```python
from build123d import *

# Parameters (mm, degrees)
SKETCH1_R            = 15
BOSS_EXTRUDE1_DEPTH  = 30
SKETCH8_W            = 30
SKETCH8_H            = 15
REVOLVE1_ANGLE       = 180
SKETCH9_W            = 30
SKETCH9_H            = 30
BOSS_EXTRUDE3_DEPTH  = 15
SKETCH10_R           = 5
CUT_EXTRUDE1_DEPTH   = 30
SKETCH13_R           = 16
CUT_EXTRUDE2_DEPTH   = 10
SKETCH14_W           = 10
SKETCH14_H           = 15
CUT_EXTRUDE3_DEPTH   = 67
CUT_EXTRUDE4_START   = -7
SKETCH15_R           = 11
SKETCH15_R_2         = 5
CUT_EXTRUDE4_DEPTH   = 7
SKETCH16_R           = 11
SKETCH16_R_2         = 5
CUT_EXTRUDE5_DEPTH   = 7
SKETCH17_R           = 15
SKETCH17_R_2         = 8
SKETCH17_R_3         = 3.5
BOSS_EXTRUDE4_DEPTH  = 2
BOSS_EXTRUDE5_DEPTH  = 5
BOSS_EXTRUDE6_DEPTH  = 16
SKETCH21_W           = 53
SKETCH21_H           = 30
CUT_EXTRUDE7_DEPTH   = 20
SKETCH23_W           = 15
SKETCH23_H           = 9
SKETCH24_W           = 30
SKETCH24_H           = 9
BOSS_EXTRUDE7_DEPTH  = 15
SKETCH25_R           = 4
CUT_EXTRUDE8_DEPTH   = 15
BOSS_EXTRUDE8_START  = 3
SKETCH26_W           = 10
SKETCH26_H           = 15
BOSS_EXTRUDE8_DEPTH  = 5
SKETCH30_W           = 30
SKETCH30_H           = 15
BOSS_EXTRUDE9_DEPTH  = 3
SKETCH27_R           = 16
CUT_EXTRUDE9_DEPTH   = 16
SKETCH28_R           = 16
CUT_EXTRUDE10_DEPTH  = 10.5
SKETCH29_R           = 16
CUT_EXTRUDE12_DEPTH  = 10
SKETCH31_W           = 53
SKETCH31_H           = 41.496728026
CUT_EXTRUDE13_DEPTH  = 37
BOSS_EXTRUDE10_DEPTH = 5
SKETCH35_W           = 30
SKETCH35_H           = 9
BOSS_EXTRUDE11_DEPTH = 5
SKETCH36_R           = 16
CUT_EXTRUDE14_DEPTH  = 13.5
SKETCH37_R           = 16
CUT_EXTRUDE15_DEPTH  = 18.5
FILLET1_R            = 5


with BuildPart() as part:
    # Sketch1 → Boss-Extrude1 (new body)
    with BuildSketch(Plane(origin=(0, 0, 0), x_dir=(1, 0, 0), z_dir=(0, 1, 0))):
        with Locations(Location((0, 0, 0), (0, 0, 270))):
            Circle(SKETCH1_R)
    extrude(amount=BOSS_EXTRUDE1_DEPTH)

    # Sketch8 → Revolve1 (revolve)
    with BuildSketch(Plane(origin=(0, 30, 0), x_dir=(1, 0, 0), z_dir=(0, 1, 0))):
        with Locations((0, -7.5)):
            Rectangle(SKETCH8_W, SKETCH8_H)
    revolve(axis=Axis((15, 30, 0), (-1, 0, 0)), revolution_arc=REVOLVE1_ANGLE)

    # Sketch9 → Boss-Extrude3 (add)
    with BuildSketch(Plane.XZ.offset(-30)):
        Rectangle(SKETCH9_W, SKETCH9_H)
    extrude(amount=BOSS_EXTRUDE3_DEPTH)

    # Sketch10 → Cut-Extrude1 (cut)
    with BuildSketch(Plane(origin=(15, 0, 0), x_dir=(0, 0, -1), z_dir=(1, 0, 0))):
        with Locations((0, 30)):
            Circle(SKETCH10_R)
    extrude(amount=-CUT_EXTRUDE1_DEPTH, mode=Mode.SUBTRACT)

    # Sketch13 → Cut-Extrude2 (cut)
    with BuildSketch(Plane(origin=(5, 0, 0), x_dir=(0, 0, -1), z_dir=(1, 0, 0))):
        with Locations((0, 30)):
            Circle(SKETCH13_R)
    extrude(amount=-CUT_EXTRUDE2_DEPTH, mode=Mode.SUBTRACT)

    # Sketch14 → Cut-Extrude3 (cut)
    with BuildSketch(Plane.XY.offset(15)):
        with Locations((0, 22.5)):
            Rectangle(SKETCH14_W, SKETCH14_H)
    extrude(amount=-CUT_EXTRUDE3_DEPTH, mode=Mode.SUBTRACT)

    # Sketch15 → Cut-Extrude4 (cut)
    with BuildSketch(Plane.ZY.offset(15).offset(CUT_EXTRUDE4_START)):
        with Locations((0, 30)):
            Circle(SKETCH15_R)
        with Locations(Location((0, 30, 0), (0, 0, 180))):
            Circle(SKETCH15_R_2, mode=Mode.SUBTRACT)
    extrude(amount=CUT_EXTRUDE4_DEPTH, mode=Mode.SUBTRACT)

    # Sketch16 → Cut-Extrude5 (cut)
    with BuildSketch(Plane(origin=(15, 0, 0), x_dir=(0, 0, -1), z_dir=(1, 0, 0))):
        with Locations(Location((0, 30, 0), (0, 0, 180))):
            Circle(SKETCH16_R)
        with Locations((0, 30)):
            Circle(SKETCH16_R_2, mode=Mode.SUBTRACT)
    extrude(amount=-CUT_EXTRUDE5_DEPTH, mode=Mode.SUBTRACT)



with BuildPart() as body_2:
    # Sketch17 → Boss-Extrude4 (new body)
    # profile 1 of 4: a face of its own
    with BuildSketch(Plane.ZY.offset(31)):
        with Locations((0, 30)):
            Circle(SKETCH17_R)
        with Locations((0, 30)):
            Circle(SKETCH17_R_2, mode=Mode.SUBTRACT)
    # profile 2 of 4: a face of its own
    with BuildSketch(Plane.ZY.offset(31)):
        with Locations((0, 30)):
            Circle(SKETCH17_R_2)
        with Locations((0, 30)):
            Circle(SKETCH17_R_3, mode=Mode.SUBTRACT)
    # profile 3 of 4: a face of its own
    with BuildSketch(Plane.ZY.offset(31)):
        with BuildLine():
            ThreePointArc((0, 15), (-10.606601718, 19.393398282), (-15, 30))
            Line((-15, 30), (-15, 15))
            Line((-15, 15), (0, 15))
        make_face()
    # profile 4 of 4: a face of its own
    with BuildSketch(Plane.ZY.offset(31)):
        with BuildLine():
            Line((15, 15), (15, 30))
            ThreePointArc((15, 30), (10.606601718, 19.393398282), (0, 15))
            Line((0, 15), (15, 15))
        make_face()
    extrude(amount=BOSS_EXTRUDE4_DEPTH)

    # Sketch18 → Boss-Extrude5 (add)
    with BuildSketch(Plane.ZY.offset(33)):
        with BuildLine():
            ThreePointArc((-8.5, 30), (0, 38.5), (8.5, 30))
            Line((8.5, 30), (8.5, 15))
            Line((8.5, 15), (15, 15))
            Line((15, 15), (15, 30))
            ThreePointArc((15, 30), (0, 45), (-15, 30))
            Line((-15, 30), (-15, 15))
            Line((-15, 15), (-8.5, 15))
            Line((-8.5, 15), (-8.5, 30))
        make_face()
    extrude(amount=BOSS_EXTRUDE5_DEPTH)


with BuildPart() as part_1:
    add(part.part)

    add(body_2.part)  # Boss-Extrude6 merges body 2
    # Sketch20 → Boss-Extrude6 (add)
    with BuildSketch(Plane.ZY.offset(15)):
        with BuildLine():
            ThreePointArc((11.5, 30), (0, 18.5), (-11.5, 30))
            Line((-11.5, 30), (-15, 30))
            Line((-15, 30), (-15, 15))
            Line((-15, 15), (0, 15))
            Line((0, 15), (15, 15))
            Line((15, 15), (15, 30))
            Line((15, 30), (11.5, 30))
        make_face()
    extrude(amount=BOSS_EXTRUDE6_DEPTH)

    # Sketch21 → Cut-Extrude7 (cut)
    with BuildSketch(Plane.XZ.offset(-15)):
        with Locations((-11.5, 0)):
            Rectangle(SKETCH21_W, SKETCH21_H)
    extrude(amount=CUT_EXTRUDE7_DEPTH, mode=Mode.SUBTRACT)


with BuildPart() as cut_extrude7_piece_1:
    # of the separate pieces the step leaves, piece 1, a body of its own (cut_extrude7_pieces)
    add(part_1.part.solids().sort_by_distance((-31, 30, 15))[0])



with BuildPart() as cut_extrude7_piece_2:
    # of the separate pieces the step leaves, piece 2, a body of its own (cut_extrude7_pieces)
    add(part_1.part.solids().sort_by_distance((5, 15, -15))[0])


with BuildPart() as body_3:
    # Sketch23 → Revolve2 (revolve)
    with BuildSketch(Plane(origin=(0, 0, 0), x_dir=(-1, 0, 0), z_dir=(0, -1, 0)), mode=Mode.PRIVATE) as revolve2_sk:
        with Locations((-7.5, 0)):
            Rectangle(SKETCH23_W, SKETCH23_H)
    revolve(revolve2_sk.sketch.rotate(Axis((0, 0, 4.5), (0, 0, -1)), 90), axis=Axis((0, 0, 4.5), (0, 0, -1)))


with BuildPart() as cut_extrude7_piece_1_1:
    add(cut_extrude7_piece_1.part)

    add(cut_extrude7_piece_2.part)  # Boss-Extrude7 merges Cut-Extrude7 piece 2

    add(body_3.part)  # Boss-Extrude7 merges body 3
    # Sketch24 → Boss-Extrude7 (add)
    with BuildSketch(Plane.XZ.offset(-15)):
        Rectangle(SKETCH24_W, SKETCH24_H)
    extrude(amount=BOSS_EXTRUDE7_DEPTH)

    # Sketch25 → Cut-Extrude8 (cut)
    with BuildSketch(Plane.XY.offset(4.5)):
        Circle(SKETCH25_R)
    extrude(amount=-CUT_EXTRUDE8_DEPTH, mode=Mode.SUBTRACT)



with BuildPart() as body_2_2:
    # Sketch26 → Boss-Extrude8 (new body)
    with BuildSketch(Plane(origin=(0, 0, -15), x_dir=(-1, 0, 0), z_dir=(0, 0, -1)).offset(BOSS_EXTRUDE8_START)):
        with Locations((-10, 22.5)):
            Rectangle(SKETCH26_W, SKETCH26_H)
        with BuildLine():
            Line((15, 30), (-5, 30))
            Line((-5, 30), (-5, 15))
            Line((-5, 15), (-12.5, 15))
            ThreePointArc((-12.5, 15), (-8.964466094, 13.535533906), (-7.5, 10))
            Line((-7.5, 10), (-7.5, 0))
            ThreePointArc((-7.5, 0), (0, 7.5), (7.5, 0))
            Line((7.5, 0), (7.5, 10))
            ThreePointArc((7.5, 10), (8.964466094, 13.535533906), (12.5, 15))
            Line((12.5, 15), (15, 15))
            Line((15, 15), (15, 30))
        make_face()
        with BuildLine():
            ThreePointArc((7.5, 0), (0, 7.5), (-7.5, 0))
            Line((-7.5, 0), (-3, 0))
            ThreePointArc((-3, 0), (0, 3), (3, 0))
            Line((3, 0), (7.5, 0))
        make_face()
        with BuildLine():
            Line((-3, 0), (-7.5, 0))
            ThreePointArc((-7.5, 0), (0, -7.5), (7.5, 0))
            Line((7.5, 0), (3, 0))
            ThreePointArc((3, 0), (0, -3), (-3, 0))
        make_face()
    extrude(amount=BOSS_EXTRUDE8_DEPTH)


with BuildPart() as cut_extrude7_piece_1_2:
    add(cut_extrude7_piece_1_1.part)

    add(body_2_2.part)  # Boss-Extrude9 merges body 2 2
    # Sketch30 → Boss-Extrude9 (add)
    with BuildSketch(Plane.XY.offset(-18)):
        with Locations((0, 22.5)):
            Rectangle(SKETCH30_W, SKETCH30_H)
    extrude(amount=BOSS_EXTRUDE9_DEPTH)

    # Sketch27 → Cut-Extrude9 (cut)
    with BuildSketch(Plane.XY.offset(4.5)):
        Circle(SKETCH27_R)
    extrude(amount=CUT_EXTRUDE9_DEPTH, mode=Mode.SUBTRACT)

    # Sketch28 → Cut-Extrude10 (cut)
    with BuildSketch(Plane(origin=(0, 0, -4.5), x_dir=(-1, 0, 0), z_dir=(0, 0, -1))):
        Circle(SKETCH28_R)
    extrude(amount=CUT_EXTRUDE10_DEPTH, mode=Mode.SUBTRACT)

    # Sketch29 → Cut-Extrude12 (cut)
    with BuildSketch(Plane.ZY.offset(-5)):
        with Locations((0, 30)):
            Circle(SKETCH29_R)
    extrude(amount=CUT_EXTRUDE12_DEPTH, mode=Mode.SUBTRACT)

    # Sketch31 → Cut-Extrude13 (cut)
    with BuildSketch(Plane.XZ.offset(-15)):
        with Locations((-11.5, -5.748364013)):
            Rectangle(SKETCH31_W, SKETCH31_H)
    extrude(amount=-CUT_EXTRUDE13_DEPTH, mode=Mode.SUBTRACT)


with BuildPart() as cut_extrude13_piece_1:
    # of the separate pieces the step leaves, piece 1, a body of its own (cut_extrude13_pieces)
    add(cut_extrude7_piece_1_2.part.solids().sort_by_distance((5, 14.645847467, 4.5))[0])



with BuildPart() as cut_extrude13_piece_2:
    # of the separate pieces the step leaves, piece 2, a body of its own (cut_extrude13_pieces)
    add(cut_extrude7_piece_1_2.part.solids().sort_by_distance((-7.5, 10, -18))[0])


with BuildPart() as cut_extrude13_piece_1_1:
    add(cut_extrude13_piece_1.part)

    add(cut_extrude13_piece_2.part)  # Boss-Extrude10 merges Cut-Extrude13 piece 2
    # Sketch33 → Boss-Extrude10 (add)
    with BuildSketch(Plane(origin=(0, 15, 0), x_dir=(1, 0, 0), z_dir=(0, 1, 0))):
        with BuildLine():
            Line((12.5, 23), (-12.5, 23))
            Line((-12.5, 23), (-12.5, 18))
            Line((-12.5, 18), (-15, 4.5))
            Line((-15, 4.5), (-15, 0))
            ThreePointArc((-15, 0), (0, -15), (15, 0))
            Line((15, 0), (15, 4.5))
            Line((15, 4.5), (12.5, 18))
            Line((12.5, 18), (12.5, 23))
        make_face()
    extrude(amount=BOSS_EXTRUDE10_DEPTH)

    # Sketch35 → Boss-Extrude11 (add)
    with BuildSketch(Plane.XZ.offset(-15)):
        Rectangle(SKETCH35_W, SKETCH35_H)
    extrude(amount=BOSS_EXTRUDE11_DEPTH)

    # Sketch36 → Cut-Extrude14 (cut)
    with BuildSketch(Plane(origin=(0, 0, -4.5), x_dir=(-1, 0, 0), z_dir=(0, 0, -1))):
        Circle(SKETCH36_R)
    extrude(amount=CUT_EXTRUDE14_DEPTH, mode=Mode.SUBTRACT)

    # Sketch37 → Cut-Extrude15 (cut)
    with BuildSketch(Plane.XY.offset(4.5)):
        Circle(SKETCH37_R)
    extrude(amount=CUT_EXTRUDE15_DEPTH, mode=Mode.SUBTRACT)

    # Fillet1
    fillet1_edges = [cut_extrude13_piece_1_1.edges().sort_by_distance(p)[0] for p in [
        (-8.964466094, 13.535533906, -23),
        (8.964466094, 13.535533906, -23),
        (7.5, 5, -23),
        (-7.5, 5, -23),
    ]]
    fillet(fillet1_edges, radius=FILLET1_R - 0.0001)  # a hair under: the kernel refuses the full size


solid = cut_extrude13_piece_1_1.part
```
For this review, take the finished solid that the model builds, in its own axes (mm). A direction names the side the tool comes from. Give positions to 0.01 mm unless a question says otherwise; leave off trailing zeros. Order: outer loops, then holes, each group sorted by start corner. A loop starts at its lowest first (then second) coordinate and runs counter-clockwise, first axis right, second up.
1) For faces 1 (the face through (0, 16, -11)), 2 (the face through (12.5, 18, -20)), 3 (the face through (-9, 15, 8)), 4 (the face through (-9, 15, -11)), list the 3-axis set-ups (+Z, -Z, +X, -X, +Y, -Y) from which the entire face can be reached by the end or side of a thin tool; tool diameter is ignored.
2) Wall thickness on line 1 (Y direction, x = 0, z = 2.5); line 2 (Z direction, x = 1.5, y = 8.5); line 3 (X direction, y = 0, z = -2.25): over which ranges is each line inside the solid? List them lowest first.
3) Insertion check: pin 1 (1.5 mm diameter, centred on y = 1, z = -18, fed in from +X); pin 2 (4 mm diameter, centred on y = 14.5, z = -19, fed in from -X); pin 3 (1.5 mm diameter, centred on y = 16.5, z = -19.5, fed in from +X); pin 4 (5 mm diameter, centred on x = 0, y = 0, fed in from +Z). Each pin has a flat end and moves straight along its axis. Give the tip position at first contact, or say it passes through.
4) Take a section at C-C (x = 13). Give the boundary of the cut face in (y, z).
5) Take a section at B-B (z = -6.5). Give the boundary of the cut face in (x, y), then the cut area to 3 significant figures.
6) Take a section at D-D (y = -1.5). State how many separate pieces and enclosed holes the cut face has, then the cut area to 3 significant figures.
7) The part is to be moulded in two halves that separate along X. For faces 5 (the face through (0, 13, -23)), 6 (the face through (0, 16, 10)), 7 (the face through (-13.732, 17.465, -11.344)), 8 (the face through (0, 17, 15)), say which applies: released by +X, released by -X, zero draft, split by the parting line, or undercut.
Derived:
1. face 1: -Y
1. face 2: -Z, +X, +Y, -Y
1. face 3: +Z, +X, -X, -Y
1. face 4: +X, -X, -Y
2. line 1: y = -15 to -4, 4 to 20
2. line 2: z = -23 to -18, -4.5 to 4.5
2. line 3: x = -15 to -4, 4 to 15
3. pin 1: stops at x = 7.5
3. pin 2: stops at x = -12.67
3. pin 3: stops at x = 12.5
3. pin 4: passes through
4. outline: (-7.48, -4.5) - (15, -4.5) - (15, -15.3) - (20, -15.3) - (20, 7.48) - (15, 7.48) - (15, 4.5) - (-7.48, 4.5) - close
5. outline: (-14.63, 15) - (-5.57, 15) arc R16 cw to (5.57, 15) - (14.63, 15) - (14.63, 20) - (-14.63, 20) - close
5. area: 139 mm2
6. separate pieces: 4
6. enclosed holes: 0
6. area: 239 mm2
7. face 5: zero draft
7. face 6: undercut
7. face 7: released by -X
7. face 8: split by the parting line
